Could you check a few things on this model? Use its own coordinates, in mm. Round coordinates to 2 decimals unless told otherwise and drop trailing zeros. Loops run counter-clockwise (first coordinate to the right, second up) from the corner with the lowest first, then second, coordinate; pieces in that order, holes last. Notation, with made-up numbers: (-31, -12.5) -> (20, -12.5) arc R25 cw to (20, 12.5) -> close; hole circle Ø2 at (6.5, 27.5). An arc over 180 degrees is marked (long way). Put each result on its own line as item: value. Start each with the question number.
1. I'm going to push flat-ended pins straight in: P1, Ø2, axis at x = 22, z = -8.5, coming from the +Y side; P2, Ø18, axis at x = 12.3, y = -347.93, coming from the -Z side; P3, Ø10, axis at x = 3, z = 4.5, coming from the +Y side. Where does each tip first touch, or does it pass through?
2. If we mould it in two halves opening along X, with no side actions, what happens to faces 1 (the cylindrical face through (29.89, -362.98, -0.17)), 2 (the cylindrical face through (10.53, 194.14, 0.18)), 3 (the cylindrical face through (-5.29, -362.98, 0.17))? For each: pulls with the +X half, pulls with the -X half, needs draft (parallel to the pull), parting line crosses it, or undercut.
3. I need wall thicknesses on line 1 (Y direction, x = 12.7, z = 1.5); line 2 (Y direction, x = 9, z = -8.75); line 3 (Y direction, x = 32.5, z = -9.5). Which ranges of each line are inside material? Lowest first, please. Write a range as [from, to].
4. Imagine slicing it at A-A, the plane z = 8.25. Please give me the cut outline in (x, y), and give its area (3 significant figures).
```python
from build123d import *

# Parameters (mm, degrees)
SKETCH7_W           = 50
SKETCH7_H           = 600
BOSS_EXTRUDE1_DEPTH = 12.5
FILLET1_R           = 27
SKETCH8_R           = 10
CUT_EXTRUDE1_DEPTH  = 375.030958071
SKETCH9_R           = 10
CUT_EXTRUDE2_DEPTH  = 375.030958071


with BuildPart() as part:
    # Sketch7 → Boss-Extrude1 (new, symmetric)
    with BuildSketch(Plane.XY):
        with Locations((12.3, -71.4)):
            Rectangle(SKETCH7_W, SKETCH7_H)
    extrude(amount=BOSS_EXTRUDE1_DEPTH, both=True)

    # Fillet1
    # the kernel refuses this fillet: 27 mm, written as the material it takes off along each edge
    with BuildSketch(Plane(origin=(37.3, -371.4, -80), x_dir=(-1, 0, 0), z_dir=(0, 0, 1)), Plane(origin=(-12.7, -371.4, 80), x_dir=(1, 0, 0), z_dir=(0, 0, -1))) as fillet1_piece_1:
        with BuildLine():
            CenterArc((FILLET1_R, -FILLET1_R), FILLET1_R, 90, 90)
            Line((0, -FILLET1_R), (0, 0))
            Line((0, 0), (FILLET1_R, 0))
        make_face()
    extrude(amount=160, mode=Mode.SUBTRACT)
    with BuildSketch(Plane(origin=(-12.7, 228.6, 80), x_dir=(1, 0, 0), z_dir=(0, 0, -1)), Plane(origin=(37.3, 228.6, -80), x_dir=(-1, 0, 0), z_dir=(0, 0, 1))) as fillet1_piece_2:
        with BuildLine():
            CenterArc((FILLET1_R, FILLET1_R), FILLET1_R, 180, 90)
            Line((0, FILLET1_R), (0, 0))
            Line((0, 0), (FILLET1_R, 0))
        make_face()
    extrude(amount=160, mode=Mode.SUBTRACT)

    # Sketch8 → Cut-Extrude1 (cut, through all)
    with BuildSketch(Plane.XY.offset(12.5)):
        with Locations((12.7, 203.901138173)):
            Circle(SKETCH8_R)
    extrude(amount=-CUT_EXTRUDE1_DEPTH, mode=Mode.SUBTRACT)

    # Sketch9 → Cut-Extrude2 (cut, through all)
    with BuildSketch(Plane.XY.offset(12.5)):
        with Locations((12.3, -347.928194148)):
            Circle(SKETCH9_R)
    extrude(amount=-CUT_EXTRUDE2_DEPTH, mode=Mode.SUBTRACT)


solid = part.part
```
Entries:
1. P1: y = 226.39
1. P2: through
1. P3: y = 227.85
2. face 1: pulls with the +X half
2. face 2: undercut
2. face 3: pulls with the -X half
3. line 1: [-371.29, -357.92], [-337.94, 193.9], [213.9, 228.49]
3. line 2: [-370.87, -357.37], [-338.49, 194.61], [213.19, 228.07]
3. line 3: [-359.77, 216.97]
4. outline: (-12.7, -344.4) arc R27 ccw to (12.3, -371.33) arc R27 ccw to (37.3, -344.4) -> (37.3, 201.6) arc R27 ccw to (12.3, 228.53) arc R27 ccw to (-12.7, 201.6) -> close; hole circle Ø20 at (12.3, -347.93); hole circle Ø20 at (12.7, 203.9)
4. area: 28,700 mm^2
